For this review, take the finished solid that the model builds, in its own axes (mm). A direction names the side the tool comes from. Give positions to 0.01 mm unless a question says otherwise; leave off trailing zeros. Order: outer loops, then holes, each group sorted by start corner. A loop starts at its lowest first (then second) coordinate and runs counter-clockwise, first axis right, second up. Notation, with made-up numbers: (-28, -16) - (-2, -16) arc R9 cw to (-2, -6) - close; hole circle Ø2 at (-31.75, 33). An arc over 180 degrees is marked (long way). Answer as a JSON object with one key per item and string values. Group by question number.
from build123d import *

# Parameters (mm, degrees)
F0_R     = 7
F0_R_2   = 2.75
F1_DEPTH = 49
F2_DEPTH = 1
F3_R     = 0.3


with BuildPart() as f1:
    # F0 (on Front) → F1 (new body)
    with BuildSketch(Plane.XZ):
        Circle(F0_R)
        Circle(F0_R_2, mode=Mode.SUBTRACT)
        Circle(F0_R_2)
    extrude(amount=-F1_DEPTH)

    # F0 (on Front) → F2 (join)
    with BuildSketch(Plane.XZ):
        Circle(F0_R_2)
    extrude(amount=F2_DEPTH)

    # F3
    f3_edges = [f1.edges().sort_by_distance(p)[0] for p in [
        (-2.75, -1, 0),
        (-7, 0, 0),
    ]]
    fillet(f3_edges, radius=F3_R)


solid = f1.part
1) Consider section A-A (y = 12.5). Give the boundary of the cut face in (x, z).
2) For faces 1 (the face through (-0.596, -0.345, -2.685)), 2 (the face through (0, 49, 0)), list the 3-axis set-ups (+Z, -Z, +X, -X, +Y, -Y) from which the entire face can be reached by the end or side of a thin tool; tool diameter is ignored.
3) For pin 1 (1.5 mm diameter, centred on x = 1, z = 5, fed in from -Y); pin 2 (3 mm diameter, centred on y = 8, z = 2, fed in from +X); pin 3 (3 mm diameter, centred on y = 27, z = -4.5, fed in from -X), all flat-tipped, find the tip position at first contact; note any pin that passes through.
4) For line 1 (Y direction, x = 3.5, z = -4.75); line 2 (Z direction, x = -2, y = 35.5); line 3 (Z direction, x = -2.75, y = 42.5), list the stretches that pass through material, from the lowest coordinate up.
Result set:
{
 "1": {"outline": "circle Ø14 at (0, 0)"},
 "2": {"face 1": "-Y", "face 2": "+Z, -Z, +X, -X, +Y"},
 "3": {"pin 1": "stops at y = 0", "pin 2": "stops at x = 6.98", "pin 3": "stops at x = -6.32"},
 "4": {"line 1": "y = 0 to 49", "line 2": "z = -6.71 to 6.71", "line 3": "z = -6.44 to 6.44"}
}
